Here's how the part is built. I have some questions about the finished solid (model axes, mm). Face numbers are marked on the shaded views. Coordinates: 2 decimals unless noted, no trailing zeros. Write each loop counter-clockwise with the first axis right and the second up, starting at its lowest first coordinate (ties: lowest second). Pieces come first, ordered by that corner, then holes. Notation, with made-up numbers: (31.25, 82) -> (44.25, 82) arc R21 ccw to (44.25, 108) -> close; hole circle Ø4 at (77.25, 37.5). An arc over 180 degrees is marked (long way). Use CSV: the item, a comma, the result in double quotes. Start each with the question number.
```python
from build123d import *

# Parameters (mm, degrees)
CROQUIS2_R              = 50
SALIENTE_EXTRUIR3_DEPTH = 30
CORTAR_EXTRUIR1_DEPTH   = 5
CORTAR_EXTRUIR2_DEPTH   = 5
CROQUIS7_R              = 15
SALIENTE_EXTRUIR4_DEPTH = 40
CROQUIS7_2_R            = 15
SALIENTE_EXTRUIR5_DEPTH = 40
CROQUIS8_R              = 7.5
CORTAR_EXTRUIR3_DEPTH   = 101


with BuildPart() as part:
    # Croquis2 → Saliente-Extruir3 (new body)
    with BuildSketch(Plane(origin=(0, 0, 0), x_dir=(1, 0, 0), z_dir=(0, 1, 0))):
        with BuildLine():
            Line((-147.4451574, 30), (-12.474701449, 58.688856044))
            ThreePointArc((-12.474701449, 58.688856044), (60, 0), (-12.474701449, -58.688856044))
            Line((-12.474701449, -58.688856044), (-147.4451574, -30))
            Line((-147.4451574, -30), (-147.4451574, 30))
        make_face()
        Circle(CROQUIS2_R, mode=Mode.SUBTRACT)
        with BuildLine():
            Line((-137.4451574, -21.902159668), (-69.084440585, -36.432678588))
            ThreePointArc((-69.084440585, -36.432678588), (-64.13537775, -34.658954459), (-63.508556655, -29.439144545))
            ThreePointArc((-63.508556655, -29.439144545), (-70, 0), (-63.508556655, 29.439144545))
            ThreePointArc((-63.508556655, 29.439144545), (-64.13537775, 34.658954459), (-69.084440585, 36.432678588))
            Line((-69.084440585, 36.432678588), (-137.4451574, 21.902159668))
            Line((-137.4451574, 21.902159668), (-137.4451574, -21.902159668))
        make_face(mode=Mode.SUBTRACT)
    extrude(amount=SALIENTE_EXTRUIR3_DEPTH)

    # Croquis4 → Cortar-Extruir1 (cut)
    with BuildSketch(Plane(origin=(0, 0, 0), x_dir=(1, 0, 0), z_dir=(0, 1, 0))):
        with BuildLine():
            Line((-147.4451574, -30), (-12.474701449, -58.688856044))
            ThreePointArc((-12.474701449, -58.688856044), (-60, 0), (-12.474701449, 58.688856044))
            Line((-12.474701449, 58.688856044), (-147.4451574, 30))
            Line((-147.4451574, 30), (-147.4451574, -30))
        make_face()
        with BuildLine():
            Line((-69.084440585, 36.432678588), (-137.4451574, 21.902159668))
            Line((-137.4451574, 21.902159668), (-137.4451574, -21.902159668))
            Line((-137.4451574, -21.902159668), (-69.084440585, -36.432678588))
            ThreePointArc((-69.084440585, -36.432678588), (-64.13537775, -34.658954459), (-63.508556655, -29.439144545))
            ThreePointArc((-63.508556655, -29.439144545), (-70, 0), (-63.508556655, 29.439144545))
            ThreePointArc((-63.508556655, 29.439144545), (-64.13537775, 34.658954459), (-69.084440585, 36.432678588))
        make_face(mode=Mode.SUBTRACT)
    extrude(amount=CORTAR_EXTRUIR1_DEPTH, mode=Mode.SUBTRACT)

    # Croquis5 → Cortar-Extruir2 (cut)
    with BuildSketch(Plane(origin=(0, 30, 0), x_dir=(1, 0, 0), z_dir=(0, 1, 0))):
        with BuildLine():
            Line((-147.4451574, 30), (-147.4451574, -30))
            Line((-147.4451574, -30), (-12.474701449, -58.688856044))
            ThreePointArc((-12.474701449, -58.688856044), (-60, 0), (-12.474701449, 58.688856044))
            Line((-12.474701449, 58.688856044), (-147.4451574, 30))
        make_face()
        with BuildLine():
            Line((-137.4451574, -21.902159668), (-69.084440585, -36.432678588))
            ThreePointArc((-69.084440585, -36.432678588), (-64.13537775, -34.658954459), (-63.508556655, -29.439144545))
            ThreePointArc((-63.508556655, -29.439144545), (-70, 0), (-63.508556655, 29.439144545))
            ThreePointArc((-63.508556655, 29.439144545), (-64.13537775, 34.658954459), (-69.084440585, 36.432678588))
            Line((-69.084440585, 36.432678588), (-137.4451574, 21.902159668))
            Line((-137.4451574, 21.902159668), (-137.4451574, -21.902159668))
        make_face(mode=Mode.SUBTRACT)
    extrude(amount=-CORTAR_EXTRUIR2_DEPTH, mode=Mode.SUBTRACT)

    # Croquis7 → Saliente-Extruir4 (add)
    with BuildSketch(Plane.XY):
        with Locations((-160, 15)):
            Circle(CROQUIS7_R)
    extrude(amount=SALIENTE_EXTRUIR4_DEPTH)

    # Croquis7<2> → Saliente-Extruir5 (add)
    with BuildSketch(Plane.XY):
        with Locations((-160, 15)):
            Circle(CROQUIS7_2_R)
    extrude(amount=-SALIENTE_EXTRUIR5_DEPTH)

    # Croquis8 → Cortar-Extruir3 (cut, through all)
    with BuildSketch(Plane.XY.offset(40)):
        with Locations((-160, 15)):
            Circle(CROQUIS8_R)
    extrude(amount=-CORTAR_EXTRUIR3_DEPTH, mode=Mode.SUBTRACT)


solid = part.part
```
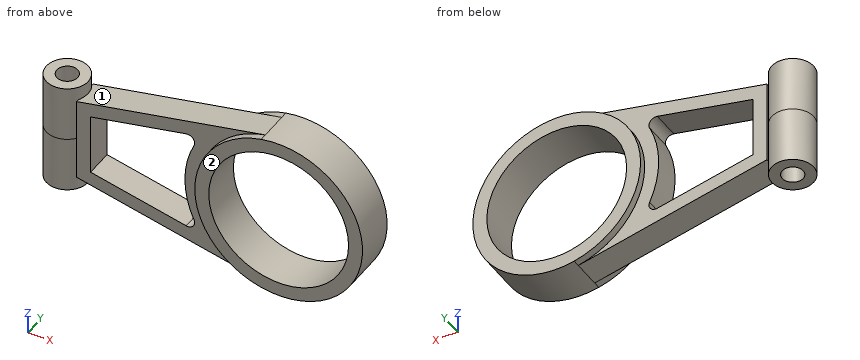
Item 1: I want a section at B-B on y = 2.25. Please give me the cut outline in (x, z).
Item 2: Thinking about a two-plate mould opening in X: for the marked faces 1 and 2, which applies, +X half, -X half, draft (parallel to the pull), parting line (faces both ways), or undercut?
Item 3: I'm going to push flat-ended pins straight in: pin 1 (5 mm diameter, centred on x = -47, y = 22.5, fed in from -Z); pin 2 (9 mm diameter, centred on x = -153, y = 18.5, fed in from +Z); pin 3 (4 mm diameter, centred on y = 8, z = -29, fed in from -X). Where does each tip first touch, or does it pass through?
Item 4: I want a section at A-A on z = 9.5. Please give me the cut outline in (x, y), then the cut area to 3 significant figures.
Item 5: If I drill on line 1 along X through (y, z) = (14.25, 0); line 2 along Y through (x, z) = (-160, 22); line 3 along X through (y, z) = (28, -34.5), over which ranges is the centre line in solid material (lowest first)?
Item 6: I want a section at D-D on y = 19.25. Please give me the cut outline in (x, z).
Item 7: I want a section at C-C on x = 0. Please give me the cut outline in (y, z).
Geometry says:
1,outline,"(-167.9, -40) -> (-152.1, -40) -> (-152.1, 40) -> (-167.9, 40) -> close; circle Ø120 at (0, 0); hole circle Ø100 at (0, 0)"
2,face 1,"undercut"
2,face 2,"draft"
3,pin 1,"z = -51.88"
3,pin 2,"z = 40"
3,pin 3,"x = -174.14"
4,outline,"(-147.45, 5) -> (-137.45, 5) -> (-137.45, 25) -> (-147.45, 25) -> (-147.45, 23.21) arc R15 ccw (long way) to (-147.45, 6.79) -> close; (-69.35, 5) -> (-59.24, 5) -> (-59.24, 0) -> (-49.09, 0) -> (-49.09, 30) -> (-59.24, 30) -> (-59.24, 25) -> (-69.35, 25) -> close; (49.09, 0) -> (59.24, 0) -> (59.24, 30) -> (49.09, 30) -> close; hole circle Ø15 at (-160, 15)"
4,area,"1,510 mm2"
5,line 1,"-174.98 to -167.46, -152.54 to -137.45, -70 to -50, 50 to 60"
5,line 2,"0 to 7.5, 22.5 to 30"
5,line 3,"-167.48 to -152.52, -49.09 to -36.19, 36.19 to 49.09"
6,outline,"(-174.39, -40) -> (-166.18, -40) -> (-166.18, 40) -> (-174.39, 40) -> close; (-153.82, -40) -> (-145.61, -40) -> (-145.61, -30.39) -> (-12.47, -58.69) arc R60 ccw (long way) to (-12.47, 58.69) -> (-145.61, 30.39) -> (-145.61, 40) -> (-153.82, 40) -> close; hole (-137.45, -21.9) -> (-69.08, -36.43) arc R5 ccw to (-63.51, -29.44) arc R70 cw to (-63.51, 29.44) arc R5 ccw to (-69.08, 36.43) -> (-137.45, 21.9) -> close; hole circle Ø100 at (0, 0)"
7,outline,"(0, -60) -> (30, -60) -> (30, -50) -> (0, -50) -> close; (0, 50) -> (30, 50) -> (30, 60) -> (0, 60) -> close"
